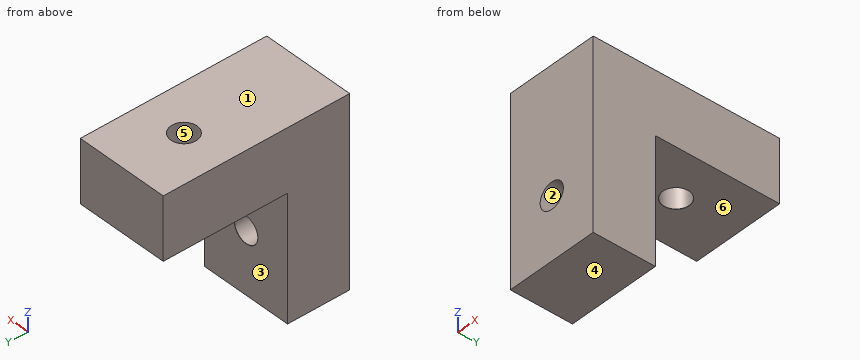
```python
from build123d import *

# Parameters (mm, degrees)
BOSS_EXTRUDE2_DEPTH                   = 15
TAP_DRILL_FOR_M5X0_8_TAP3_D           = 4.2
TAP_DRILL_FOR_M5X0_8_TAP3_CSINK_D     = 4.25
TAP_DRILL_FOR_M5X0_8_TAP3_CSINK_ANGLE = 90
TAP_DRILL_FOR_M5X0_8_TAP4_D           = 4.2
TAP_DRILL_FOR_M5X0_8_TAP4_CSINK_D     = 4.25
TAP_DRILL_FOR_M5X0_8_TAP4_CSINK_ANGLE = 90


with BuildPart() as part:
    # Sketch8 → Boss-Extrude2 (new body)
    with BuildSketch(Plane(origin=(0, 0, 0), x_dir=(0, 0, -1), z_dir=(1, 0, 0))):
        Polygon((0, 30), (0, 0), (30, 0), (30, 10), (10, 10), (10, 30), align=None)
    extrude(amount=BOSS_EXTRUDE2_DEPTH)

    # Tap Drill for M5x0.8 Tap3 (through all)
    with Locations(Plane(origin=(0, 10, 0), x_dir=(1, 0, 0), z_dir=(0, 1, 0))):
        with Locations((7.5, 20)):
            CounterSinkHole(TAP_DRILL_FOR_M5X0_8_TAP3_D / 2, TAP_DRILL_FOR_M5X0_8_TAP3_CSINK_D / 2, counter_sink_angle=TAP_DRILL_FOR_M5X0_8_TAP3_CSINK_ANGLE)

    # Tap Drill for M5x0.8 Tap4 (through all)
    with Locations(Plane(origin=(0, 0, -10), x_dir=(-1, 0, 0), z_dir=(0, 0, -1))):
        with Locations((-7.5, 20)):
            CounterSinkHole(TAP_DRILL_FOR_M5X0_8_TAP4_D / 2, TAP_DRILL_FOR_M5X0_8_TAP4_CSINK_D / 2, counter_sink_angle=TAP_DRILL_FOR_M5X0_8_TAP4_CSINK_ANGLE)


solid = part.part
```
Read the model definition and answer for the solid it produces. Units are mm, in the model's axes. Face numbers are marked on the shaded views. A direction names the side the tool comes from. Coordinates: 2 decimals unless noted, no trailing zeros. Loops run counter-clockwise (first coordinate to the right, second up) from the corner with the lowest first, then second, coordinate; pieces in that order, holes last. Notation, with made-up numbers: (-1, 75.5) -> (9, 75.5) arc R24 ccw to (9, 103.5) -> close; hole circle Ø10 at (-22.5, -27.75). An arc over 180 degrees is marked (long way). Return JSON: item names as keys, results as strings.
Item 1: Find section B-B (x = 7.5). Determine the outline of the cut face in (y, z) (3 decimals).
Answers:
{"outline": "(0, -30) -> (10, -30) -> (10, -22.125) -> (9.975, -22.1) -> (0, -22.1) -> close; (0, -17.9) -> (9.975, -17.9) -> (10, -17.875) -> (10, -10) -> (17.875, -10) -> (17.9, -9.975) -> (17.9, 0) -> (0, 0) -> close; (22.1, -9.975) -> (22.125, -10) -> (30, -10) -> (30, 0) -> (22.1, 0) -> close"}
Item 2: For a pull along Z with two mould halves and no side action, classify the marked faces 1, 2, 3 and 4 as +Z half, -Z half, draft (parallel to the pull), parting line (faces both ways), or undercut.
Answers:
{"face 1": "+Z half", "face 2": "undercut", "face 3": "draft", "face 4": "-Z half"}
Item 3: Find section A-A (z = -20). Determine the outline of the cut face in (x, y) (3 decimals), plus the area to 3 significant figures.
Answers:
{"outline": "(0, 0) -> (5.4, 0) -> (5.4, 9.975) -> (5.375, 10) -> (0, 10) -> close; (9.6, 0) -> (15, 0) -> (15, 10) -> (9.625, 10) -> (9.6, 9.975) -> close", "area": "108 mm2"}
Item 4: Find section C-C (x = 1.5). Determine the outline of the cut face in (y, z).
Answers:
{"outline": "(0, -30) -> (10, -30) -> (10, -10) -> (30, -10) -> (30, 0) -> (0, 0) -> close"}
Item 5: Find the intervals of material crossed by probe 1 along Y at (x, z) = (7.5, -6.25); probe 2 along X at (y, z) = (4, -20); probe 3 along Y at (x, z) = (8.25, -15), in increasing order.
Answers:
{"probe 1": "y = 0 to 17.9, 22.1 to 30", "probe 2": "x = 0 to 5.4, 9.6 to 15", "probe 3": "y = 0 to 10"}
Item 6: Find section D-D (y = 10.5). Determine the outline of the cut face in (x, z).
Answers:
{"outline": "(0, -10) -> (15, -10) -> (15, 0) -> (0, 0) -> close"}
Item 7: For the marked faces 5 and 6, determine the directions among +Z, -Z, +X, -X, +Y, -Y from which every point of the face is accessible in a straight line to the end or side of a thin tool.
Answers:
{"face 5": "+Z, -Z", "face 6": "-Z, +X, -X, +Y"}
Item 8: Flat-ended cylindrical pins translate along their axes: P1, Ø7.5, axis at x = 8, z = -22, coming from the +Y side; P2, Ø7.5, axis at x = 6, y = 22, coming from the -Z side; P3, Ø4, axis at x = 7.5, z = -20, coming from the -Y side. Find the tip coordinate at first contact, or state that the pin passes through.
Answers:
{"P1": "stops at y = 10", "P2": "stops at z = -10", "P3": "passes through"}
